```python
from build123d import *

# Parameters (mm, degrees)
F0_R     = 6.35
F1_DEPTH = 9.525


with BuildPart() as f1:
    # F0 (on Top) → F1 (new body)
    with BuildSketch(Plane.XY):
        with BuildLine():
            Line((63.5, 63.5), (-63.5, 63.5))
            Line((-63.5, 63.5), (-63.5, -5.625801))
            ThreePointArc((-63.5, -5.625801), (-58.966732, -22.833307), (-46.543764, -35.573741))
            Line((-46.543764, -35.573741), (-17.968764, -52.718741))
            ThreePointArc((-17.968764, -52.718741), (0, -57.695801), (17.968764, -52.718741))
            Line((17.968764, -52.718741), (46.543764, -35.573741))
            ThreePointArc((46.543764, -35.573741), (58.966732, -22.833307), (63.5, -5.625801))
            Line((63.5, -5.625801), (63.5, 63.5))
        make_face()
        with Locations((0, -32.295801)):
            Circle(F0_R, mode=Mode.SUBTRACT)
        with Locations((-47.742878, 19.05)):
            Circle(F0_R, mode=Mode.SUBTRACT)
        with Locations((42.999213, 19.05)):
            Circle(F0_R, mode=Mode.SUBTRACT)
    extrude(amount=F1_DEPTH)


solid = f1.part
```
Build history of the part. All positions in model axes, mm. Give positions to 0.01 mm unless a question says otherwise; leave off trailing zeros. Loops run counter-clockwise (first coordinate to the right, second up) from the corner with the lowest first, then second, coordinate; pieces in that order, holes last. Notation, with made-up numbers: (6, 6.5) -> (37, 6.5) arc R26 ccw to (37, 41.5) -> close; hole circle Ø7 at (6.5, -23.5). An arc over 180 degrees is marked (long way). One line per question, with ' | ' between items. Start each with the question number.
1) Pin check, flat tips, straight feed: pin 1 (4 mm diameter, centred on x = -26.5, z = 7, fed in from -Y); pin 2 (4 mm diameter, centred on x = 0.5, z = 7, fed in from -Y). Stop position of each tip, or through.
2) Cut at A-A (x = 0). Give the cut face in (y, z) (3 decimals).
3) Probe L1, parallel to Y at x = 0, z = 2.25; L2, parallel to X at y = 22, z = 5; L3, parallel to Y at x = 2, z = 1. List the from-to ranges inside material, lowest first.
4) Cut at C-C (z = 6.5). Give the cut face in (x, y) (3 decimals).
5) Cut at B-B (y = 19.05). Give the cut face in (x, z) (3 decimals).
6) Cut at D-D (y = -28). Give the cut face in (x, z) (3 decimals), plus the area to 3 significant figures.
7) Two-plate mould, pull along Y, no slides. Class faces 1 (the flat face through (32.056, -44.266, 4.696)), 2 (the flat face through (63.5, 28, 5)), 3 (the cylindrical face through (-0.83, -26, 4.7)): released by +Y, released by -Y, zero draft, split by the parting line, or undercut.
Return value:
1) pin 1: y = -48.8 | pin 2: y = -57.7
2) outline: (-57.696, 0) -> (-38.646, 0) -> (-38.646, 9.525) -> (-57.696, 9.525) -> close; (-25.946, 0) -> (63.5, 0) -> (63.5, 9.525) -> (-25.946, 9.525) -> close
3) L1: -57.7 to -38.65, -25.95 to 63.5 | L2: -63.5 to -53.37, -42.12 to 37.38, 48.62 to 63.5 | L3: -57.64 to -38.32, -26.27 to 63.5
4) outline: (-63.5, -5.626) arc R34.925 ccw to (-46.544, -35.574) -> (-17.969, -52.719) arc R34.925 ccw to (17.969, -52.719) -> (46.544, -35.574) arc R34.925 ccw to (63.5, -5.626) -> (63.5, 63.5) -> (-63.5, 63.5) -> close; hole circle Ø12.7 at (-47.743, 19.05); hole circle Ø12.7 at (0, -32.296); hole circle Ø12.7 at (42.999, 19.05)
5) outline: (-63.5, 0) -> (-54.093, 0) -> (-54.093, 9.525) -> (-63.5, 9.525) -> close; (-41.393, 0) -> (36.649, 0) -> (36.649, 9.525) -> (-41.393, 9.525) -> close; (49.349, 0) -> (63.5, 0) -> (63.5, 9.525) -> (49.349, 9.525) -> close
6) outline: (-55.392, 0) -> (-4.676, 0) -> (-4.676, 9.525) -> (-55.392, 9.525) -> close; (4.676, 0) -> (55.392, 0) -> (55.392, 9.525) -> (4.676, 9.525) -> close | area: 966 mm^2
7) face 1: released by -Y | face 2: zero draft | face 3: undercut
